Autodesk Inventor part; units mm, degrees
ref_plane "YZ Plane" through (0, 0, 0) normal (1, 0, 0) x (0, 1, 0)
ref_plane "XZ Plane" through (0, 0, 0) normal (0, 1, 0) x (-1, 0, 0)
ref_plane "XY Plane" through (0, 0, 0) normal (0, 0, 1) x (1, 0, 0)
sketch "Skizze1" plane through (0, 0, 0) normal (0, 0, 1) x (1, 0, 0)
  line L0 (-3, 1.5) -> (1.5, 1.5)
  line L1 (1.5, 1.5) -> (1.5, -1.5)
  line L2 (-3, -1.5) -> (-3, 1.5)
  line L3 (1.5, 1.5) -> (-1.5, -1.5) construction
  line L4 (-1.5, -1.5) -> (1.5, -1.5) construction
  line L5 (0, 0) -> (0.1963, -0.4081) construction
  line L6 (-3, -1.5) -> (1.5, -1.5)
  dimension "d0" = 3
  dimension "d1" = 4.5
extrude "Extrusion1" add sketch "Skizze1" against normal blind 0.75
sketch "Skizze2" plane through (0, 0, 0) normal (1, 0, 0) x (0, 1, 0)
  line L0 (-1.5, 0) -> (1.5, 0)
  arc A0 (0, 1.5) -> (-1.5, 0) centre (0, 0) ccw
  line L1 (0, 0) -> (0, 1.5)
  line L2 (0, 0) -> (-1.5, 0)
  dimension "d4" = 1.5
revolve "Umdrehung1" add sketch "Skizze2" angle 360 about axis through (0, 0, 0) along (0, 0, 1)
sketch "Skizze3" plane through (0, 0, -0.75) normal (0, 0, -1) x (-1, 0, 0)
  line L0 (11.4893, 0) -> (5.7446, -9.95)
  line L1 (5.7446, -9.95) -> (-5.7446, -9.95)
  line L2 (-5.7446, -9.95) -> (-11.4893, 0)
  line L3 (-11.4893, 0) -> (-5.7446, 9.95)
  line L4 (-5.7446, 9.95) -> (5.7446, 9.95)
  line L5 (5.7446, 9.95) -> (11.4893, 0)
  point P0 (0, 0)
  point P1 (0, 0)
  dimension "d7" = 19.9
extrude "Extrusion2" add sketch "Skizze3" along normal blind 1.8
sketch "Skizze4" plane through (0, 0, -0.75) normal (0, 0, 1) x (1, 0, 0)
  line L0 (-11.4893, 0) -> (-5.7446, -9.95)
  line L1 (-5.7446, 9.95) -> (-11.4893, 0)
  line L2 (1.5, -1.5) -> (-3, -1.5)
  line L3 (0, 0) -> (-9.77, 0) construction
  arc A0 (-9.77, -1.5) -> (-9.77, 1.5) centre (-9.77, 0) ccw
  line L4 (-9.77, -1.5) -> (-10.6232, -1.5)
  line L5 (-9.77, 1.5) -> (-10.6232, 1.5)
  dimension "d10" = 9.77
  dimension "d11" = 3
extrude "Extrusion3" cut sketch "Skizze4" against normal blind 1.8
pattern_circular "Runde Anordnung1" count 6 over 360 about axis through (0, 0, -10) along (0, 0, 1) of "Extrusion3"
properties part number "Luxeon Rebel Star"
Work out the finished part from the listing and answer in its coordinate system (mm). A direction names the side the tool comes from. Give positions to 0.01 mm unless a question says otherwise; leave off trailing zeros. Loops run counter-clockwise (first coordinate to the right, second up) from the corner with the lowest first, then second, coordinate; pieces in that order, holes last. Notation, with made-up numbers: (50.5, 67.25) - (101.5, 67.25) arc R11 ccw to (101.5, 82.25) - close; hole circle Ø1 at (48, -35). An arc over 180 degrees is marked (long way). Answer in a Markdown table with one row per item. Add a question column.
Q1. The part is cut by section A-A (x = -2). Determine the outline of the cut face in (y, z).
Q2. The part is cut by section C-C (y = 6.5). Determine the outline of the cut face in (x, z), and give its area (3 significant figures).
Q3. Each of these flat-tipped pins is pushed along its axis until it touches: P1, Ø10, axis at x = -7.5, y = 3, coming from the +Z side; P2, Ø0.6, axis at y = 0, z = 0, coming from the +X side; P3, Ø0.6, axis at x = 0, z = -0.5, coming from the +Y side; P4, Ø1.5, axis at x = -1, y = 0, coming from the +Z side. Where does it stop, or does it pass through?
Q4. A tool of negligible diameter and unlimited length cuts with its end or side. For faces 1 (the flat face through (-10, 1.5, -2)), 2 (the flat face through (1.14, 1.2, 0)), 3 (the flat face through (8.59, -5.02, -1.64)), 4 (the flat face through (10, 1.5, -2)), 5 (the flat face through (1.2, -1.2, 0)), from which of +Z, -Z, +X, -X, +Y, -Y can it reach the whole face along a straight path? Write none if from no direction.
Q5. The part is cut by section D-D (x = 4.5). Determine the outline of the cut face in (y, z), and give its area (3 significant figures).
Q6. The part is cut by section B-B (z = -1.3). Determine the outline of the cut face in (x, y) (3 decimals), and give its area (3 significant figures).
Q7. Consider line 1 along X through (y, z) = (-8.5, -0.8); line 2 along Z through (x, y) = (1.25, -8.75); line 3 along Y through (x, z) = (-1, -0.3). Determine where each line is inside the solid, lowest interval first.
Q8. Determine the mould class of faces 6 (the cylindrical face through (8.27, 0.03, -1.64)), 7 (the cylindrical face through (-4.16, 7.15, -1.64)), 8 (the flat face through (-2, 0, 0)) for opening direction X: released by +X, released by -X, zero draft, split by the parting line, or undercut.
Solution:
| question | item | result |
|---|---|---|
| 1 | outline | (-9.95, -2.55) - (9.95, -2.55) - (9.95, -0.75) - (1.5, -0.75) - (1.5, 0) - (-1.5, 0) - (-1.5, -0.75) - (-9.95, -0.75) - close |
| 2 | outline | (-7.74, -2.55) - (7.74, -2.55) - (7.74, -0.75) - (-7.74, -0.75) - close |
| 2 | area | 27.9 mm² |
| 3 | P1 | stops at z = 0 |
| 3 | P2 | stops at x = 1.5 |
| 3 | P3 | stops at y = 9.95 |
| 3 | P4 | stops at z = 1.48 |
| 4 | face 1 | +Z, -Z, -X |
| 4 | face 2 | +Z, +X, +Y |
| 4 | face 3 | +Z, -Z, +X, -Y |
| 4 | face 4 | +Z, -Z, +X |
| 4 | face 5 | +Z, +X, -Y |
| 5 | outline | (-7.01, -2.55) - (7.01, -2.55) - (7.01, -0.75) - (-7.01, -0.75) - close |
| 5 | area | 25.2 mm² |
| 6 | outline | (-10.623, -1.5) - (-6.611, -8.45) - (-6.184, -7.711) arc R1.5 cw to (-3.586, -9.211) - (-4.013, -9.95) - (4.013, -9.95) - (3.586, -9.211) arc R1.5 cw to (6.184, -7.711) - (6.611, -8.45) - (10.623, -1.5) - (9.77, -1.5) arc R1.5 cw to (9.77, 1.5) - (10.623, 1.5) - (6.611, 8.45) - (6.184, 7.711) arc R1.5 cw to (3.586, 9.211) - (4.013, 9.95) - (-4.013, 9.95) - (-3.586, 9.211) arc R1.5 cw to (-6.184, 7.711) - (-6.611, 8.45) - (-10.623, 1.5) - (-9.77, 1.5) arc R1.5 cw to (-9.77, -1.5) - close |
| 6 | area | 299 mm² |
| 7 | line 1 | x = -3.39 to 3.39 |
| 7 | line 2 | z = -2.55 to -0.75 |
| 7 | line 3 | y = -1.5 to 1.5 |
| 8 | face 6 | released by +X |
| 8 | face 7 | undercut |
| 8 | face 8 | zero draft |
